Autodesk Fusion 360 part; units mm, degrees
sketch "スケッチ1" plane through (0, 0, 0) normal (0, 0, 1) x (1, 0, 0)
  line L0 (0, 0) -> (148.1, 0)
  line L1 (148.1, 0) -> (148.1, 40)
  line L2 (148.1, 40) -> (0, 40)
  line L3 (0, 40) -> (0, 0)
  dimension "d1" = 148.1
  dimension "d2" = 40
extrude "押し出し1" add sketch "スケッチ1" along normal blind 8.8
sketch "スケッチ2" plane through (0, 0, 8.8) normal (0, 0, 1) x (-1, 0, 0)
  line L0 (0, -40) -> (0, 0)
  line L1 (0, 0) -> (-148.1, 0)
  line L2 (-148.1, 0) -> (-148.1, -40)
  line L3 (-148.1, -40) -> (0, -40)
  line L4 (-148.1, -40) -> (-102.2, -40)
  line L5 (-102.2, -40) -> (-102.2, -33.5)
  line L6 (-102.2, -33.5) -> (-148.1, -33.5)
  line L7 (-148.1, -33.5) -> (-148.1, -40)
  line L8 (-148.1, 0) -> (-102.2, 0)
  line L9 (-102.2, 0) -> (-102.2, -6.5)
  line L10 (-102.2, -6.5) -> (-148.1, -6.5)
  line L11 (-148.1, -6.5) -> (-148.1, 0)
  line L12 (0, -40) -> (-59.9, -40)
  line L13 (-59.9, -40) -> (-59.9, -34.5)
  line L14 (-59.9, -34.5) -> (0, -34.5)
  line L15 (0, -34.5) -> (0, -40)
  line L16 (0, 0) -> (-59.9, 0)
  line L17 (-59.9, 0) -> (-59.9, -5.5)
  line L18 (-59.9, -5.5) -> (0, -5.5)
  line L19 (0, -5.5) -> (0, 0)
  line L20 (-59.9, -40) -> (-102.2, -40)
  line L21 (-102.2, -40) -> (-102.2, 0)
  line L22 (-102.2, 0) -> (-59.9, 0)
  line L23 (-59.9, 0) -> (-59.9, -40)
  dimension "d5" = 45.9
  dimension "d6" = 6.5
  dimension "d7" = 45.9
  dimension "d8" = 6.5
  dimension "d9" = 59.9
  dimension "d10" = 5.5
  dimension "d11" = 59.9
  dimension "d12" = 5.5
extrude "押し出し2" add sketch "スケッチ2" along normal blind 11.2 contours L0 L3 L12 L13 L14 L15 L23 | L1 L3 L5 L9 L13 L17 L20 L21 L22 L23 | L0 L1 L16 L17 L18 L19 L23 | L2 L3 L4 L5 L6 L7 L21 | L1 L2 L8 L9 L10 L11 L21
extrude "押し出し5" cut 1 faces at (117.5, 24.5, 8.8) along direction (0, 0, -1) blind 1.8
sketch "スケッチ4" plane through (0, 0, 7) normal (0, 0, 1) x (-1, 0, 0)
  line L0 (-102.2, -6.5) -> (-148.1, -6.5)
  line L1 (-148.1, -6.5) -> (-148.1, -33.5)
  line L2 (-148.1, -33.5) -> (-102.2, -33.5)
  line L3 (-102.2, -33.5) -> (-102.2, -6.5)
  line L4 (-148.1, -33.5) -> (-143.1, -33.5)
  line L5 (-143.1, -33.5) -> (-143.1, -6.5)
  line L6 (-143.1, -6.5) -> (-148.1, -6.5)
  line L7 (-148.1, -6.5) -> (-148.1, -33.5)
  dimension "d22" = 5
extrude "押し出し6" add sketch "スケッチ4" along normal blind 3.8 contours L0 L1 L2 L4 L5 L6 L7
sketch "スケッチ7" plane through (102.2, 0, 0) normal (1, 0, 0) x (0, 1, 0)
  line L0 (33.5, 7) -> (33.5, 20)
  line L1 (33.5, 20) -> (6.5, 20)
  line L2 (6.5, 20) -> (6.5, 7)
  line L3 (6.5, 7) -> (33.5, 7)
  circle A0 centre (20, 20) radius 18
  dimension "d28" = 36
extrude "押し出し8" cut sketch "スケッチ7" against normal blind 42.3 contours L0 L1 L2 L3 A0 | L0 L1 L2 A0 | L3 A0
sketch "スケッチ8" plane through (0, 0, 10.8) normal (0, 0, 1) x (-1, 0, 0)
  line L0 (-148.1, -6.5) -> (-148.1, -33.5)
  line L1 (-148.1, -33.5) -> (-143.1, -33.5)
  line L2 (-143.1, -33.5) -> (-143.1, -6.5)
  line L3 (-143.1, -6.5) -> (-148.1, -6.5)
  line L4 (-144.5, -32.5) -> (-146.1, -32.5)
  line L5 (-146.1, -32.5) -> (-146.1, -28.5)
  line L6 (-146.1, -28.5) -> (-144.5, -28.5)
  line L7 (-144.5, -28.5) -> (-144.5, -32.5)
  line L8 (-146.1, -7.5) -> (-144.5, -7.5)
  line L9 (-144.5, -7.5) -> (-144.5, -11.5)
  line L10 (-144.5, -11.5) -> (-146.1, -11.5)
  line L11 (-146.1, -11.5) -> (-146.1, -7.5)
  dimension "d31" = 1.6
  dimension "d32" = 4
  dimension "d33" = 1.4
  dimension "d34" = 1
  dimension "d35" = 1.6
  dimension "d36" = 4
  dimension "d37" = 1
  dimension "d38" = 1.4
extrude "押し出し9" cut sketch "スケッチ8" against normal blind 4 contours L4 L5 L6 L7 | L8 L9 L10 L11
sketch "スケッチ9" plane through (148.1, 0, 0) normal (1, 0, 0) x (0, 1, 0)
  line L0 (33.5, 20) -> (33.5, 10.8)
  line L1 (33.5, 10.8) -> (6.5, 10.8)
  line L2 (6.5, 10.8) -> (6.5, 20)
  line L3 (6.5, 20) -> (0, 20)
  line L4 (0, 20) -> (0, 0)
  line L5 (0, 0) -> (40, 0)
  line L6 (40, 0) -> (40, 20)
  line L7 (40, 20) -> (33.5, 20)
  circle A0 centre (9.5, 9) radius 1.05
  circle A1 centre (30.5, 9) radius 1.05
  point P0 (30.5, 9)
  point P1 (9.5, 9)
  dimension "d41" = 9.5
  dimension "d42" = 1.8
  dimension "d43" = 9.5
  dimension "d44" = 1.8
  dimension "d45" = 2.1
  dimension "d46" = 2.1
extrude "押し出し10" cut sketch "スケッチ9" against normal blind 5 contours A0 | A1
sketch "スケッチ10" plane through (148.1, 0, 0) normal (1, 0, 0) x (0, 1, 0)
  circle A0 centre (9.5, 9) radius 1.05
  circle A1 centre (30.5, 9) radius 1.05
  line L0 (33.5, 20) -> (33.5, 10.8)
  line L1 (33.5, 10.8) -> (6.5, 10.8)
  line L2 (6.5, 10.8) -> (6.5, 20)
  line L3 (6.5, 20) -> (0, 20)
  line L4 (0, 20) -> (0, 0)
  line L5 (0, 0) -> (40, 0)
  line L6 (40, 0) -> (40, 20)
  line L7 (40, 20) -> (33.5, 20)
  line L8 (12.5, 10.8) -> (27.5, 10.8)
  line L9 (27.5, 10.8) -> (27.5, 7)
  line L10 (27.5, 7) -> (12.5, 7)
  line L11 (12.5, 7) -> (12.5, 10.8)
  dimension "d49" = 15
  dimension "d50" = 3.8
  dimension "d51" = 12.5
extrude "押し出し11" cut sketch "スケッチ10" against normal blind 1 contours L1 L8 L9 L10 L11
The model under review builds one solid part; all positions refer to its coordinate system, in mm. A direction names the side the tool comes from. Round coordinates to 2 decimals unless told otherwise and drop trailing zeros. Loops run counter-clockwise (first coordinate to the right, second up) from the corner with the lowest first, then second, coordinate; pieces in that order, holes last. Notation, with made-up numbers: M 73,21.25 L 82,21.25 A33 ccw 82,54.25 Z; hole C 43,7.5 d4. An arc over 180 degrees is marked long. Answer as CSV lines item,"result".
1. We need section C-C (z = 18.5). Give the boundary of the cut face in (x, y), plus the area to 3 significant figures.
Outcome:
outline,"M 0,0 L 148.1,0 L 148.1,6.5 L 102.2,6.5 L 102.2,2.06 L 59.9,2.06 L 59.9,5.5 L 0,5.5 Z; M 0,34.5 L 59.9,34.5 L 59.9,37.94 L 102.2,37.94 L 102.2,33.5 L 148.1,33.5 L 148.1,40 L 0,40 Z"
area,"1,430 mm2"
2. We need section A-A (y = 20). Give the boundary of the cut face in (x, z), plus the area to 3 significant figures.
Outcome:
outline,"M 0,0 L 148.1,0 L 148.1,7 L 147.1,7 L 147.1,10.8 L 143.1,10.8 L 143.1,7 L 102.2,7 L 102.2,2 L 59.9,2 L 59.9,8.8 L 0,8.8 Z"
area,"948 mm2"
3. Insertion check: pin 1 Ø2 at (y, z) = (16.5, 11.5) entering from -X; pin 2 Ø2.5 at (x, y) = (145.5, 24.5) entering from +Z. Each pin has a flat end and moves straight along its axis. Give the tip position at first contact, or say it passes through.
Outcome:
pin 1,"stops at x = 143.1"
pin 2,"stops at z = 10.8"
4. To check wall thickness, follow L1, parallel to X at y = 30, z = 8; L2, parallel to Z at x = 146.9, y = 30.5; L3, parallel to X at y = 17.5, z = 8. State the ranges of each line that lie inside material, in increasing order. Write a range as [from, to].
Outcome:
L1,"x = [0, 59.9], [143.1, 144.5], [146.1, 148.1]"
L2,"z = [0, 7.95], [10.05, 10.8]"
L3,"x = [0, 59.9], [143.1, 147.1]"
5. We need section D-D (z = 4.75). Give the boundary of the cut face in (x, y), plus the area to 3 significant figures.
Outcome:
outline,"M 0,0 L 148.1,0 L 148.1,40 L 0,40 Z; hole M 59.9,10.44 L 102.2,10.44 L 102.2,29.56 L 59.9,29.56 Z"
area,"5,120 mm2"
6. For faces 5 (the face through (30, 34.5, 14)), 6 (the face through (59.9, 4, 16)), 7 (the face through (75, 39, 20)), list the 3-axis set-ups (+Z, -Z, +X, -X, +Y, -Y) from which the entire face can be reached by the end or side of a thin tool; tool diameter is ignored.
Outcome:
face 5,"+Z, -X"
face 6,"+Z"
face 7,"+Z, +X, -X, +Y, -Y"
7. We need section B-B (x = 134). Give the boundary of the cut face in (y, z).
Outcome:
outline,"M 0,0 L 40,0 L 40,20 L 33.5,20 L 33.5,7 L 6.5,7 L 6.5,20 L 0,20 Z"
8. Draft analysis for pull direction Y (two halves, no side actions). For faces 1 (the face through (73, 0, 10)), 2 (the face through (146, 20, 10.8)), 3 (the face through (73, 20, 0)), 4 (the face through (146.1, 10, 7.9)), state which applies: pulls with the +Y half, pulls with the -Y half, needs draft (parallel to the pull), parting line crosses it, or undercut.
Outcome:
face 1,"pulls with the -Y half"
face 2,"undercut"
face 3,"needs draft"
face 4,"undercut"
